Drawing for the job (mm, zero at the part's lowest x, y, z). A direction names the side the tool comes from. Round coordinates to 2 decimals unless told otherwise and drop trailing zeros. Loops run counter-clockwise (first coordinate to the right, second up) from the corner with the lowest first, then second, coordinate; pieces in that order, holes last.
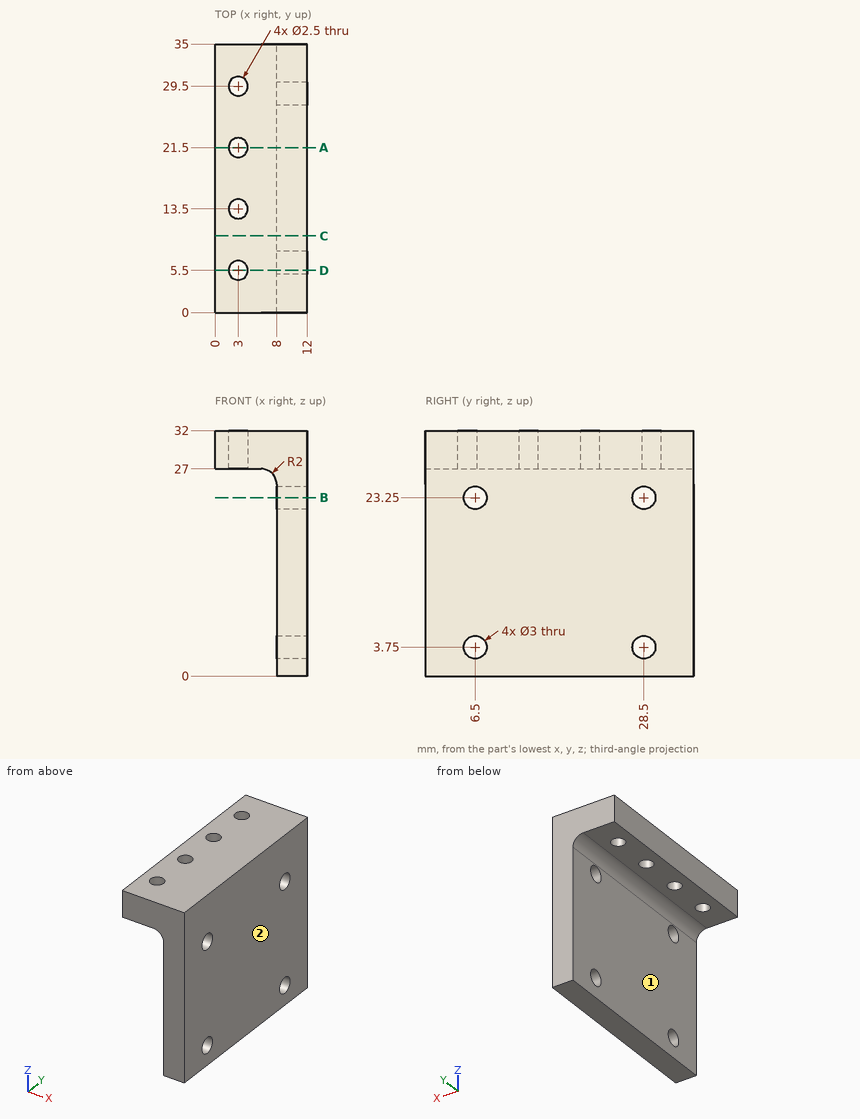
Q1. Slice it at B-B on z = 23.25. Give the cut face in (x, y), plus the area to 3 significant figures.
Q2. Probe line 1 (Y direction, x = 10.9, z = 3.75); line 2 (X direction, y = 25, z = 4); line 3 (Y direction, x = 2.25, z = 30.5). List the from-to ranges inside material, lowest first.
Q3. Slice it at A-A on y = 21.5. Give the cut face in (x, z), plus the area to 3 significant figures.
Q4. Tool access for the marked faces 1 and 2: list every direction of +Z, -Z, +X, -X, +Y, -Y with a clear straight run to the whole face (end or side of a thin tool).
Q5. Slice it at C-C on y = 10. Give the cut face in (x, z).
Q6. Flat gauge pins, fed straight in: P1, Ø10, axis at y = 22.5, z = 8, coming from the -X side; P2, Ø5, axis at x = 1.5, y = 11, coming from the -Z side. Where does each tip first touch, or does it go through?
Q7. Slice it at D-D on y = 5.5. Give the cut face in (x, z).
Reply:
1. outline: (8, 0) - (12, 0) - (12, 5) - (8, 5) - close; (8, 8) - (12, 8) - (12, 27) - (8, 27) - close; (8, 30) - (12, 30) - (12, 35) - (8, 35) - close
1. area: 116 mm2
2. line 1: y = 0 to 5, 8 to 27, 30 to 35
2. line 2: x = 8 to 12
2. line 3: y = 0 to 4.5, 6.5 to 12.5, 14.5 to 20.5, 22.5 to 28.5, 30.5 to 35
3. outline: (0, 27) - (1.75, 27) - (1.75, 32) - (0, 32) - close; (4.25, 27) - (6, 27) arc R2 cw to (8, 25) - (8, 0) - (12, 0) - (12, 32) - (4.25, 32) - close
3. area: 156 mm2
4. face 1: -Z, -X, +Y, -Y
4. face 2: +Z, -Z, +X, +Y, -Y
5. outline: (0, 27) - (6, 27) arc R2 cw to (8, 25) - (8, 0) - (12, 0) - (12, 32) - (0, 32) - close
6. P1: stops at x = 8
6. P2: stops at z = 27
7. outline: (0, 27) - (1.75, 27) - (1.75, 32) - (0, 32) - close; (4.25, 27) - (6, 27) arc R2 cw to (8, 25) - (8, 24.37) - (12, 24.37) - (12, 32) - (4.25, 32) - close; (8, 0) - (12, 0) - (12, 2.63) - (8, 2.63) - close; (8, 4.87) - (12, 4.87) - (12, 22.13) - (8, 22.13) - close
